Autodesk Inventor part; units mm, degrees
ref_plane "YZ Plane" through (0, 0, 0) normal (1, 0, 0) x (0, 1, 0)
ref_plane "XZ Plane" through (0, 0, 0) normal (0, 1, 0) x (-1, 0, 0)
ref_plane "XY Plane" through (0, 0, 0) normal (0, 0, 1) x (1, 0, 0)
sketch "スケッチ1" plane through (0, 0, 0) normal (0, 0, 1) x (1, 0, 0)
  line L0 (150, 150) -> (150, -150)
  line L1 (150, -150) -> (-150, -150)
  line L2 (-150, -150) -> (-150, 150)
  line L3 (-150, 150) -> (150, 150)
  circle A0 centre (0, 0) radius 90
  dimension "d0" = 300
  dimension "d1" = 180
extrude "押し出し1" add sketch "スケッチ1" along normal blind 15
properties part number "障害物、丸１"
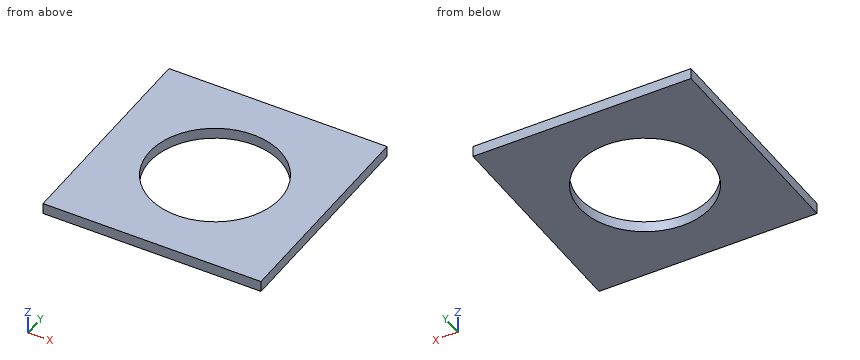
For this review, take the finished solid that the model builds, in its own axes (mm). Coordinates: 2 decimals unless noted, no trailing zeros. Loops run counter-clockwise (first coordinate to the right, second up) from the corner with the lowest first, then second, coordinate; pieces in that order, holes last. Notation, with made-up numbers: (45, -23) - (55, -23) arc R29 ccw to (55, 6) - close; hole circle Ø3 at (64.5, -11.75). An arc over 180 degrees is marked (long way). Use one line per item in the form item = value. Start each with the question number.
1) Take a section at C-C (z = 9). State the section outline as (x, y) points.
2) For pin 1 (5 mm diameter, centred on x = 41.5, y = -85.5, fed in from -Z), flat-tipped, find the tip position at first contact; note if it passes through.
3) To check wall thickness, follow probe 1 along Y at (x, z) = (0, 6); probe 2 along Y at (x, z) = (55, 13.75); probe 3 along X at (y, z) = (-30, 8.5). State the ranges of each line that lie inside material, in increasing order. Write a range as from..to.
4) Take a section at A-A (y = 0). State the section outline as (x, z) points.
From the geometry:
q1.outline = (-150, -150) - (150, -150) - (150, 150) - (-150, 150) - close; hole circle Ø180 at (0, 0)
q2.pin_1 = 0
q3.probe_1 = -150..-90, 90..150
q3.probe_2 = -150..-71.24, 71.24..150
q3.probe_3 = -150..-84.85, 84.85..150
q4.outline = (-150, 0) - (-90, 0) - (-90, 15) - (-150, 15) - close; (90, 0) - (150, 0) - (150, 15) - (90, 15) - close
